Check sheet for the modelled part. Datum: model origin and axes. Units: mm. Round coordinates to 2 decimals unless told otherwise and drop trailing zeros. Order: outer loops, then holes, each group sorted by start corner. A loop starts at its lowest first (then second) coordinate and runs counter-clockwise, first axis right, second up. Notation, with made-up numbers: (66.5, 17.5) -> (84.5, 17.5) arc R15 ccw to (84.5, 40.5) -> close; hole circle Ø5 at (-29.75, -34.5). An arc over 180 degrees is marked (long way). Answer in a Markdown table with one row per item.
Autodesk Inventor part; units mm, degrees
ref_plane "Work Plane2" through (0, 0, 10) normal (0, 0, 1) x (1, 0, 0)
ref_plane "YZ Plane" through (0, 0, 0) normal (1, 0, 0) x (0, 1, 0)
ref_plane "XZ Plane" through (0, 0, 0) normal (0, 1, 0) x (-1, 0, 0)
sketch "Sketch1" plane through (0, 0, 0) normal (1, 0, 0) x (0, 1, 0)
  line L0 (8.7312, 8.7312) -> (-8.7312, 8.7312)
  line L1 (-8.7312, 8.7312) -> (-8.7313, -8.7313)
  line L2 (-8.7313, -8.7313) -> (8.7312, -8.7313)
  line L3 (8.7312, -8.7313) -> (8.7312, 8.7312)
  line L4 (8.7312, 8.7312) -> (-8.7313, -8.7313) construction
  line L5 (-8.7312, 8.7312) -> (8.7312, -8.7313) construction
  point P0 (0, 0)
  point P1 (0, 0)
  dimension "d9" = 17.4625
  dimension "d10" = 17.4625
extrude "Extrusion1" add sketch "Sketch1" against normal blind 425
ref_plane "Work Plane2" through (0, 0, 10) normal (0, 0, 1) x (1, 0, 0)
sketch "Sketch2" plane through (0, 0, 0) normal (0, 0, 1) x (1, 0, 0)
  circle A0 centre (-125, 0) radius 3.175
  line L0 (0, 8.7312) -> (0, -8.7312) construction
  line L1 (-425, 8.7312) -> (-425, -8.7313) construction
  point P0 (0, 0)
  dimension "d7" = 6.35
  dimension "d11" = 300
extrude "Extrusion2" add sketch "Sketch2" along normal mid plane 80
sketch "Sketch4" plane through (0, -8.7312, 8.7312) normal (0, 0, 1) x (1, 0, 0)
  circle A0 centre (-125, 8.7312) radius 3.175 construction
  point P0 (0, 8.7312)
  point P1 (-5, 8.7312)
  dimension "d14" = 120
hole "Hole1" at (-5, 0, 8.7312) direction (0, 0, -1) diameter 5 end through all
sketch "Sketch3" plane through (-125, 0, 40) normal (0, 0, 1) x (1, 0, 0)
  circle A0 centre (0, 0) radius 3.175
  line L0 (-300, -8.7312) -> (-300, 8.7312) construction
  line L1 (125, 8.7312) -> (125, -8.7312) construction
  point P0 (125, 0)
  dimension "d12" = 300
  dimension "d13" = 125
equation "\"LongArmLen\" = 300"
equation "\"ShortArmLen\" = 120"
properties part number "Long Arm"
Item 1: Cross-section at A-A (x = -306). Record the boundary of the cut face in (y, z), and give its area (3 significant figures).
Result sheet:
| item | result |
|---|---|
| outline | (-8.73, -8.73) -> (8.73, -8.73) -> (8.73, 8.73) -> (-8.73, 8.73) -> close |
| area | 305 mm^2 |
Item 2: Scan lines: line 1 (X direction, y = 0, z = 4); line 2 (Y direction, x = -5, z = -1); line 3 (Z direction, x = -30, y = -6.5). Record each from-to range of solid material in increasing order. Write a range as [from, to].
Result sheet:
| item | result |
|---|---|
| line 1 | x = [-425, -7.5], [-2.5, 0] |
| line 2 | y = [-8.73, -2.5], [2.5, 8.73] |
| line 3 | z = [-8.73, 8.73] |
Item 3: Cross-section at B-B (z = -26). Record the boundary of the cut face in (x, y) (3 decimals), and give its area (3 significant figures).
Result sheet:
| item | result |
|---|---|
| outline | circle Ø6.35 at (-125, 0) |
| area | 31.7 mm^2 |
Item 4: Depth check by flat-ended pin: P1, Ø5, axis at x = -288.5, y = -1, coming from the -Z side; P2, Ø8, axis at x = -72.5, y = 1.5, coming from the +Z side. Enter the tip coordinate at first touch or a pass-through.
Result sheet:
| item | result |
|---|---|
| P1 | stops at z = -8.73 |
| P2 | stops at z = 8.73 |
